The drawing under review shows one solid part. Ordinate dimensions are in mm from its lowest x, y, z. A direction names the side the tool comes from. Give positions to 0.01 mm unless a question says otherwise; leave off trailing zeros. Loops run counter-clockwise (first coordinate to the right, second up) from the corner with the lowest first, then second, coordinate; pieces in that order, holes last. Notation, with made-up numbers: M 63.25,-20 L 88.25,-20 A9 ccw 88.25,-7 Z; hole C 5.5,58.5 d4. An arc over 180 degrees is marked long. One line per item, written item: value. Start each with the question number.
Q1. We need section D-D on y = 3.75. Write out the cut boundary in (x, z).
Q2. We need section B-B on y = 20.5. Write out the cut boundary in (x, z).
Q3. For the marked faces 1 and 2, list the 3-axis set-ups (+Z, -Z, +X, -X, +Y, -Y) from which the entire face can be reached by the end or side of a thin tool; tool diameter is ignored.
Q4. We need section A-A on z = 42. Write out the cut boundary in (x, y) (1 decimal).
Q5. For pin 1 (9.5 mm diameter, centred on x = 40.46, z = 34.95, fed in from +Y); pin 2 (2 mm diameter, centred on y = 15, z = 33.5, fed in from +X); pin 3 (12 mm diameter, centred on x = 8, y = 3.5, fed in from +Z); pin 4 (12 mm diameter, centred on y = 10.5, z = 32, fed in from -X), all flat-tipped, find the tip position at first contact; note any pin that passes through.
Q6. Mouldability with a two-part tool opening along X and no side actions: class the marked faces 3, 4 and 5 as released by +X, released by -X, zero draft, split by the parting line, or undercut.
Q7. To check wall thickness, follow line 1 along Y through (x, z) = (17, 10); line 2 along Z through (x, y) = (42, 15) (1 decimal); line 3 along Z through (x, y) = (56, 1.5). State the ranges of each line that lie inside material, in increasing order. Write a range as from..to.
Q8. We need section C-C on x = 5.5. Write out the cut boundary in (y, z), plus the area to 3 significant figures.
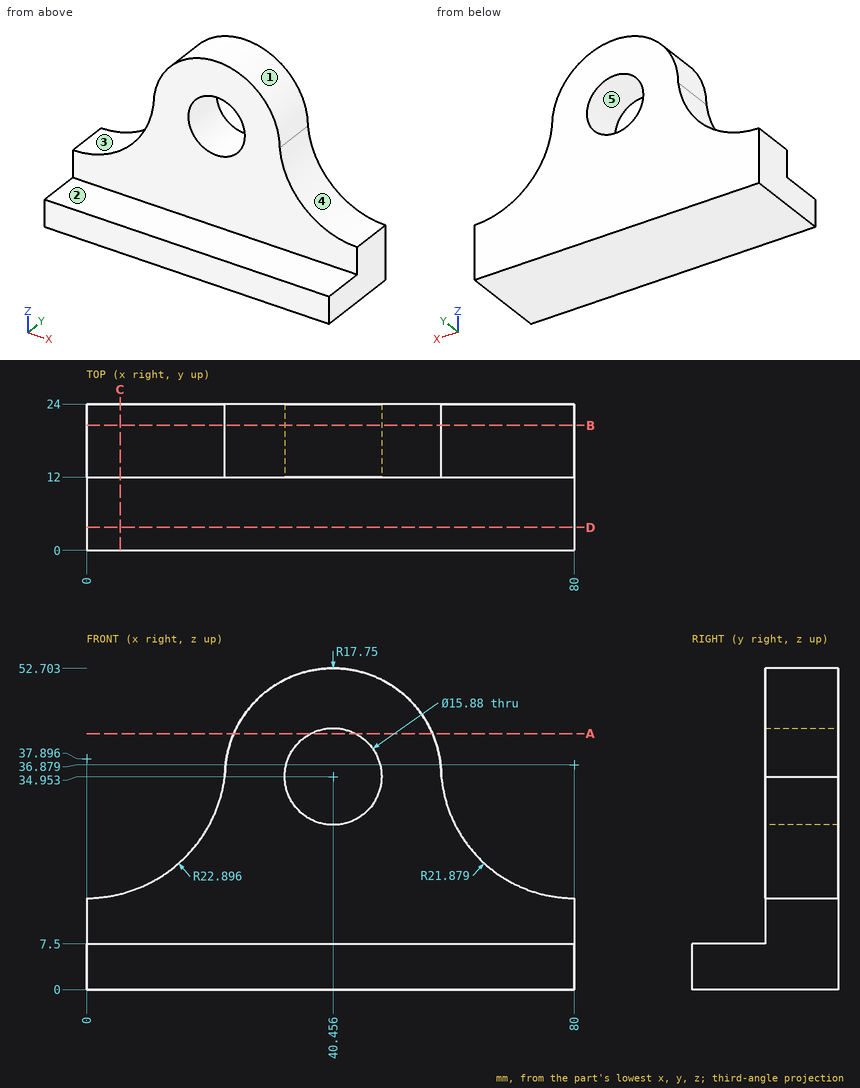
Solved:
1. outline: M 0,0 L 80,0 L 80,7.5 L 0,7.5 Z
2. outline: M 0,0 L 80,0 L 80,15 A21.88 cw 58.21,34.95 A17.75 ccw 22.71,34.95 A22.9 cw 0,15 Z; hole C 40.46,34.95 d15.88
3. face 1: +Z, +Y, -Y
3. face 2: +Z, +X, -X, -Y
4. outline: M 24.2,12 L 36.8,12 L 36.8,24 L 24.2,24 Z; M 44.1,12 L 56.7,12 L 56.7,24 L 44.1,24 Z
5. pin 1: through
5. pin 2: x = 58.56
5. pin 3: z = 7.5
5. pin 4: x = 19.68
6. face 3: released by -X
6. face 4: released by +X
6. face 5: undercut
7. line 1: 12..24
7. line 2: 0..27.2, 42.7..52.6
7. line 3: 0..7.5
8. outline: M 0,0 L 24,0 L 24,15.67 L 12,15.67 L 12,7.5 L 0,7.5 Z
8. area: 278 mm2
